Answer from the drawing. Dimensions are ordinates in mm from the lowest x, y and z of the part. A direction names the side the tool comes from. Give positions to 0.01 mm unless a question says otherwise; leave off trailing zeros. Write each loop counter-clockwise with the first axis right and the second up, starting at its lowest first coordinate (ties: lowest second). Pieces come first, ordered by that corner, then holes. Notation, with made-up numbers: (83, -11) -> (133, -11) arc R24 cw to (133, 1) -> close; hole circle Ø6 at (22, -4). An arc over 180 degrees is marked (long way). Put each result on its own line as item: value. Start each with the question number.
1) A cutting plane is placed at B-B (y = 8). Write down the section's boundary in (x, z), then the cut area to 3 significant figures.
2) Find the intervals of material crossed by line 1 along X through (y, z) = (8, 19.65); line 2 along Z through (x, y) = (12.5, 4.25), in increasing order. Write a range as from..to.
3) A cutting plane is placed at A-A (x = 10). Write down the section's boundary in (y, z).
4) A cutting plane is placed at C-C (x = 18.5). Write down the section's boundary in (y, z).
5) For the marked faces 1 and 2, determine the directions among +Z, -Z, +X, -X, +Y, -Y from which every point of the face is accessible in a straight line to the end or side of a thin tool.
6) A cutting plane is placed at D-D (y = 1.5). Write down the section's boundary in (x, z).
7) Flat-ended cylindrical pins translate along their axes: pin 1 Ø8 at (x, z) = (11, 6) entering from -Y; pin 2 Ø5 at (y, z) = (5, 14.5) entering from -X; pin 3 Ø6.5 at (x, y) = (10, 8) entering from -Z. Find the tip coordinate at first contact, or state that the pin passes through.
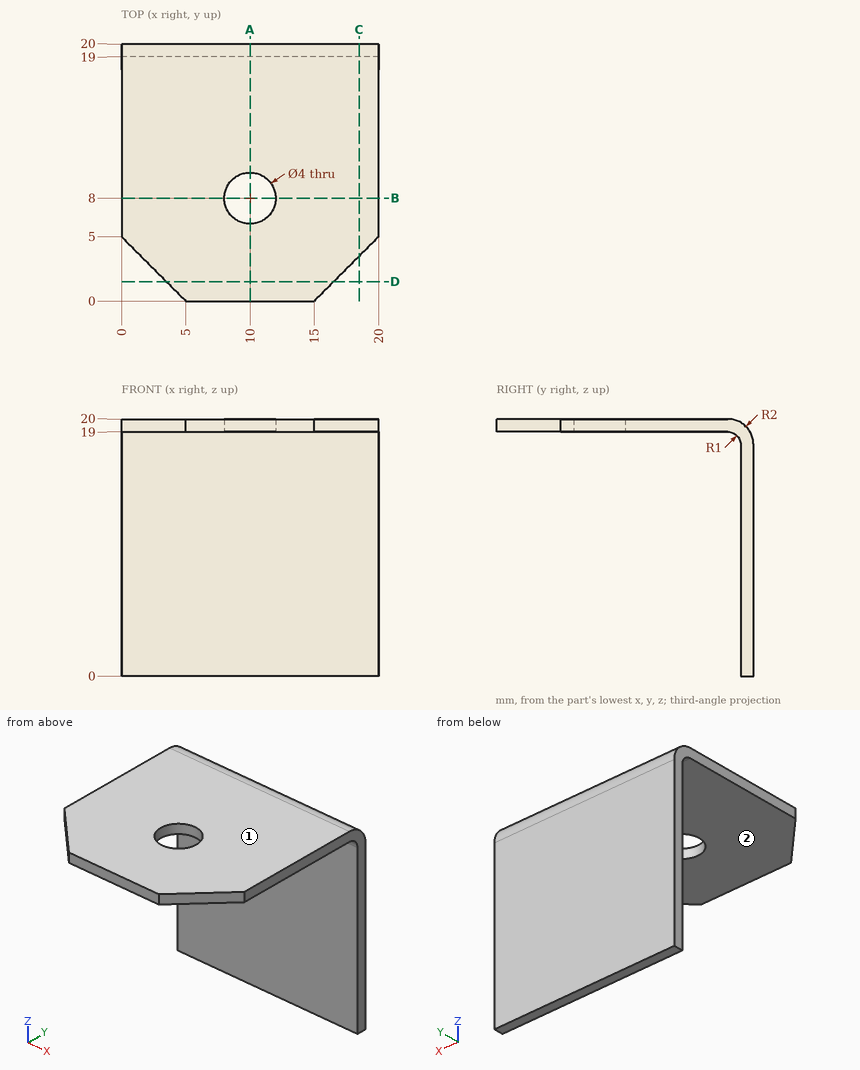
Reply:
1. outline: (0, 19) -> (8, 19) -> (8, 20) -> (0, 20) -> close; (12, 19) -> (20, 19) -> (20, 20) -> (12, 20) -> close
1. area: 16.0 mm2
2. line 1: x = 0..8, 12..20
2. line 2: z = 19..20
3. outline: (0, 19) -> (6, 19) -> (6, 20) -> (0, 20) -> close; (10, 19) -> (18, 19) arc R1 cw to (19, 18) -> (19, 0) -> (20, 0) -> (20, 18) arc R2 ccw to (18, 20) -> (10, 20) -> close
4. outline: (3.5, 19) -> (18, 19) arc R1 cw to (19, 18) -> (19, 0) -> (20, 0) -> (20, 18) arc R2 ccw to (18, 20) -> (3.5, 20) -> close
5. face 1: +Z, +X, -X, +Y, -Y
5. face 2: -Z, +X, -X, -Y
6. outline: (3.5, 19) -> (16.5, 19) -> (16.5, 20) -> (3.5, 20) -> close
7. pin 1: stops at y = 19
7. pin 2: passes through
7. pin 3: stops at z = 19
